from build123d import *

# Parameters (mm, degrees)
BOSS_EXTRUDE1_DEPTH      = 8.5
SKETCH2_W                = 17
SKETCH2_H                = 17
CUT_EXTRUDE1_DEPTH       = 6
CUT_EXTRUDE2_REACH       = 29.591
ESBO_O1_W                = 20
ESBO_O1_H                = 3
RESSALTO_EXTRUS_O1_DEPTH = 40
ESBO_O2_W                = 3
ESBO_O2_H                = 30
RESSALTO_EXTRUS_O2_DEPTH = 57
RESSALTO_EXTRUS_O3_REACH = 62.434
ESBO_O3_W                = 2.5
ESBO_O3_H                = 17
ESBO_O5_W                = 14.5
ESBO_O5_H                = 27
CORTE_EXTRUS_O1_DEPTH    = 61.433848132
CORTE_EXTRUS_O2_DEPTH    = 62.491869381
FILETE1_R                = 5
ESBO_O7_R                = 2.099999999
ESBO_O7_R_2              = 4.7
CORTE_EXTRUS_O3_DEPTH    = 62.491817705


with BuildPart() as part:
    # Sketch1 → Boss-Extrude1 (new, symmetric)
    with BuildSketch(Plane(origin=(0, 0, 0), x_dir=(0, 0, -1), z_dir=(1, 0, 0))):
        Polygon((0, 0), (-20, 0), (-20, -3), (-11.5, -11.5), (-3, -20), (0, -20), align=None)
    extrude(amount=BOSS_EXTRUDE1_DEPTH, both=True)

    # Sketch2 → Cut-Extrude1 (cut, symmetric)
    with BuildSketch(Plane(origin=(0, 0, 0), x_dir=(0, 0, -1), z_dir=(1, 0, 0))):
        with Locations((-11.5, -11.5)):
            Rectangle(SKETCH2_W, SKETCH2_H)
    extrude(amount=CUT_EXTRUDE1_DEPTH, both=True, mode=Mode.SUBTRACT)

    # Sketch3 → Cut-Extrude2 (cut, up to next)
    with BuildSketch(Plane.XY.offset(3), mode=Mode.PRIVATE) as cut_extrude2_sk1:
        with BuildLine():
            Line((-3, -9), (-3, -12))
            ThreePointArc((-3, -12), (0, -15), (3, -12))
            Line((3, -12), (3, -9))
            ThreePointArc((3, -9), (0, -6), (-3, -9))
        make_face()
    cut_extrude2_tool1 = extrude(cut_extrude2_sk1.sketch, amount=-CUT_EXTRUDE2_REACH, mode=Mode.PRIVATE) & part.part
    cut_extrude2 = cut_extrude2_tool1.solids().sort_by_distance((0, -10.5, 3))[0]
    add(cut_extrude2, mode=Mode.SUBTRACT)

    # Mirror1: Cut-Extrude2 across plane
    add(cut_extrude2.mirror(Plane(origin=(0, 0, 0), x_dir=(0, -0.7071067811865481, 0.707106781186547), z_dir=(0, 0.7071067811865471, 0.707106781186548))), mode=Mode.SUBTRACT)

    # Esboço1 → Ressalto-extrusão1 (add)
    with BuildSketch(Plane.ZY.offset(8.5)):
        with Locations((10, -1.5)):
            Rectangle(ESBO_O1_W, ESBO_O1_H)
    extrude(amount=RESSALTO_EXTRUS_O1_DEPTH)

    # Esboço2 → Ressalto-extrusão2 (add)
    with BuildSketch(Plane(origin=(8.5, 0, 0), x_dir=(0, 0, -1), z_dir=(1, 0, 0))):
        with Locations((-21.5, -15)):
            Rectangle(ESBO_O2_W, ESBO_O2_H)
    extrude(amount=-RESSALTO_EXTRUS_O2_DEPTH)

    # Ressalto-extrusão3: up to this face of the body (flat: up to its plane)
    ressalto_extrus_o3_end = Plane(part.part.faces().sort_by_distance((7.25, -11.5, 11.5))[0])
    # Esboço3 → Ressalto-extrusão3 (add, up to the picked face)
    with BuildSketch(Plane(origin=(0, 0, 20), x_dir=(-1, 0, 0), z_dir=(0, 0, -1)), mode=Mode.PRIVATE) as ressalto_extrus_o3_sk1:
        with Locations((7.25, -11.5)):
            Rectangle(ESBO_O3_W, ESBO_O3_H)
    ressalto_extrus_o3_tool1 = split(extrude(ressalto_extrus_o3_sk1.sketch, amount=RESSALTO_EXTRUS_O3_REACH, mode=Mode.PRIVATE), bisect_by=ressalto_extrus_o3_end, keep=Keep.BOTH, mode=Mode.PRIVATE)
    add(ressalto_extrus_o3_tool1.solids().sort_by(Axis((-7.25, -11.5, 20), (0, 0, -1)))[0])

    # Esboço5 → Corte-extrusão1 (cut, through all)
    with BuildSketch(Plane(origin=(0, 0, 20), x_dir=(-1, 0, 0), z_dir=(0, 0, -1))):
        with Locations((-1.25, -16.5)):
            Rectangle(ESBO_O5_W, ESBO_O5_H)
    extrude(amount=-CORTE_EXTRUS_O1_DEPTH, mode=Mode.SUBTRACT)

    # Esboço6 → Corte-extrusão2 (cut, through all)
    with BuildSketch(Plane.XY.offset(23)):
        Polygon((-48.5, -13), (-12.043382351, -30), (-48.5, -30), align=None)
    extrude(amount=-CORTE_EXTRUS_O2_DEPTH, mode=Mode.SUBTRACT)

    # Filete1
    # the kernel refuses this fillet: 5 mm, written as the material it takes off along each edge
    with BuildSketch(Plane(origin=(-48.5, -13, 30.96337826), x_dir=(0, 1, 0), z_dir=(0, 0, -1))) as filete1_piece_1:
        with BuildLine():
            CenterArc((FILETE1_R * 0.637070260807, FILETE1_R), FILETE1_R, 205, 65)
            Line((-FILETE1_R * 0.269237526229, FILETE1_R * 0.577381738259), (0, 0))
            Line((0, 0), (FILETE1_R * 0.637070260807, 0))
        make_face()
    extrude(amount=18.92675652, mode=Mode.SUBTRACT)
    with BuildSketch(Plane(origin=(-12.043382351, -30, 25.771183283), x_dir=(-0.9063077870366518, 0.4226182617406957, 0), z_dir=(0, 0, -1))) as filete1_piece_2:
        with BuildLine():
            CenterArc((FILETE1_R * 0.221694662643, FILETE1_R), FILETE1_R, 245, 25)
            Line((-FILETE1_R * 0.200923599098, FILETE1_R * 0.0936922129633), (0, 0))
            Line((0, 0), (FILETE1_R * 0.221694662643, 0))
        make_face()
    extrude(amount=8.542366566, mode=Mode.SUBTRACT)
    with BuildSketch(Plane(origin=(-6, -30, 7.5), x_dir=(-1, 0, 0), z_dir=(0, 0, 1))) as filete1_piece_3:
        with BuildLine():
            CenterArc((FILETE1_R, -FILETE1_R), FILETE1_R, 90, 90)
            Line((0, -FILETE1_R), (0, 0))
            Line((0, 0), (FILETE1_R, 0))
        make_face()
    extrude(amount=28, mode=Mode.SUBTRACT)

    # Esboço7 → Corte-extrusão3 (cut, through all)
    with BuildSketch(Plane.XY.offset(23)):
        with Locations((-42.541332366, -10.354642716)):
            Circle(ESBO_O7_R)
        with Locations((-10.82055982, -25.146281877)):
            Circle(ESBO_O7_R)
        with Locations((-23.3, -10.5)):
            Circle(ESBO_O7_R_2)
    extrude(amount=-CORTE_EXTRUS_O3_DEPTH, mode=Mode.SUBTRACT)


solid = part.part
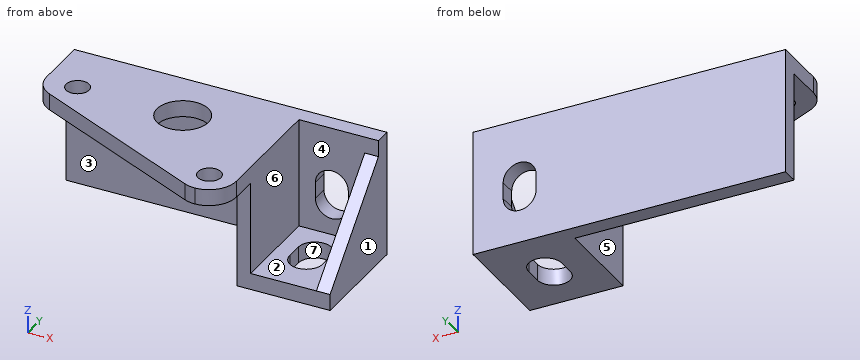
CAD build for the part. Positions are in the model's coordinates, mm. Face numbers are marked on the shaded views. A direction names the side the tool comes from. Give positions to 0.01 mm unless a question says otherwise; leave off trailing zeros. Write each loop counter-clockwise with the first axis right and the second up, starting at its lowest first coordinate (ties: lowest second). Pieces come first, ordered by that corner, then holes. Notation, with made-up numbers: (41.5, 6.5) - (98.5, 6.5) arc R21 ccw to (98.5, 12.5) - close; hole circle Ø8 at (34.5, 67.5). An arc over 180 degrees is marked (long way). Put each result on its own line as item: value.
(1) Pull direction X, two halves, no side cores. Call the marked faces 1, 2, 3 and 4: released by +X, released by -X, zero draft, split by the parting line, or undercut.
Working result:
face 1: released by +X
face 2: undercut
face 3: zero draft
face 4: undercut
(2) Tool access for the marked faces 5, 6 and 7: list every direction of +Z, -Z, +X, -X, +Y, -Y with a clear straight run to the whole face (end or side of a thin tool).
Working result:
face 5: -Z, -X, -Y
face 6: +Z, -Y
face 7: +Z, -Z
(3) Saw through at B-B (z = 21). List the corners of the cut face in (x, y), then the cut area to 3 significant figures.
Working result:
outline: (-48.5, -9.81) arc R5 ccw to (-45.61, -14.35) - (-13.05, -29.53) arc R5 ccw to (-10.97, -30) arc R5 ccw to (-6, -25) - (-6, -3) - (8.5, -3) - (8.5, 0) - (-48.5, 0) - close; hole circle Ø4.2 at (-42.54, -10.35); hole circle Ø9.4 at (-23.3, -10.5); hole circle Ø4.2 at (-10.82, -25.15)
area: 904 mm^2
(4) Drop flat-ended pins along their axis: pin 1 Ø0.9 at (y, z) = (-10.5, 1) entering from -X; pin 2 Ø3.5 at (x, y) = (0.5, -15) entering from +Z; pin 3 Ø4.5 at (x, z) = (2, 14.5) entering from -Y. Give the stop position or say it passes through.
Working result:
pin 1: x = -8.5
pin 2: z = 3
pin 3: y = -3
(5) Saw through at D-D (z = 4). List the corners of the cut face in (x, y).
Working result:
outline: (-48.5, -3) - (-8.5, -3) - (-8.5, -20) - (-6, -20) - (-6, -3) - (6, -3) - (6, -19) - (8.5, -19) - (8.5, 0) - (-48.5, 0) - close
(6) Saw through at C-C (x = -23.3). List the corners of the cut face in (y, z).
Working result:
outline: (-24.75, 20) - (-15.2, 20) - (-15.2, 23) - (-24.75, 23) - close; (-5.8, 20) - (-3, 20) - (-3, 0) - (0, 0) - (0, 23) - (-5.8, 23) - close
(7) Saw through at A-A (x = 0). List the corners of the cut face in (y, z).
Working result:
outline: (-20, 0) - (-15, 0) - (-15, 3) - (-20, 3) - close; (-6, 0) - (0, 0) - (0, 6) - (-3, 6) - (-3, 3) - (-6, 3) - close; (-3, 15) - (0, 15) - (0, 23) - (-3, 23) - close
(8) Wall check: L1, parallel to X at y = -5, z = 7.5; L2, parallel to Z at x = 0, y = -1.5; L3, parallel to Y at x = -13, z = 18.5. Give the ranges that are in metal, low to high.
Working result:
L1: -8.5 to -6, 6 to 8.5
L2: 0 to 6, 15 to 23
L3: -3 to 0
